Geometry: final body of the model. Coordinates: model frame, mm. A direction names the side the tool comes from. Coordinates: 2 decimals unless noted, no trailing zeros. Write each loop counter-clockwise with the first axis right and the second up, starting at its lowest first coordinate (ties: lowest second). Pieces come first, ordered by that corner, then holes. Notation, with made-up numbers: M 79.5,-26.75 L 113.5,-26.75 A7 ccw 113.5,-17.75 Z; hole C 62.25,10.5 d3. An arc over 180 degrees is marked long. Write item = value, one per line. Start each with the question number.
Item 1: Ray query, L1, parallel to Z at x = -27, y = -110.45; L2, parallel to Y at x = -227, z = 8.5; L3, parallel to Y at x = -419.5, z = 7.5. Return the intervals inside material, ascending. Write a range as [from, to].
Item 2: Reachability of faces 1 (the cylindrical face through (-30.23, 110.79, 18.79)), 2 (the flat face through (-62, -126.75, 25)), 3 (the flat face through (-214.22, 184.18, 24.65)) from +Z, -Z, +X, -X, +Y, -Y: full face, straight path, thin tool, end or side. Return the list, or none.
Item 3: First-contact query: pin 1 Ø6.5 at (y, z) = (-112, 17) entering from +X; pin 2 Ø12.5 at (x, z) = (-27, 25) entering from +Y; pin 3 Ø12 at (x, z) = (-290, 36.5) entering from -Y. Flat tips, straight axial feed; report the tip coordinate or a pass-through.
Item 4: Pull-direction query (Y, two-part tool) for faces 4 (the flat face through (-62, 126.75, 25)), 5 (the flat face through (-56, 120.75, 25)), 6 (the flat face through (-286.95, -242.43, 24.65)), 7 (the cylindrical face through (-23.77, -123.79, 18.79)); classes: +Y half, -Y half, draft (parallel to the pull), parting line (faces both ways), or undercut.
Item 5: Section B-B on y = 267. Output: boundary loops of the cut face in (x, z).
Item 6: Section A-A on x = -266. Output: boundary loops of the cut face in (y, z).
from build123d import *

# Parameters (mm, degrees)
PAD_DEPTH           = 50
PAD001_DEPTH        = 50
SKETCH015_R         = 6
POCKET005_DEPTH     = 10
LINEARPATTERN_COUNT = 4
LINEARPATTERN_PITCH = 130
PAD007_DEPTH        = 10
CHAMFER_SIZE        = 5
SKETCH016_R         = 7
POCKET_DEPTH        = 20
SKETCH017_R         = 7
POCKET006_DEPTH     = 20


with BuildPart() as part:
    # Sketch → Pad (new body)
    with BuildSketch(Plane.XY):
        with BuildLine():
            Line((-447.593833, 354.914912), (19.501599, 27.85117))
            ThreePointArc((34, 0), (30.158368, 15.699453), (19.501599, 27.85117))
            Line((28, 0), (34, 0))
            ThreePointArc((28, 0), (24.836303, 12.928961), (16.06014, 22.936257))
            Line((16.06014, 22.936257), (-451.035292, 350))
            Line((-451.035292, 350), (-447.593833, 354.914912))
        make_face()
    extrude(amount=PAD_DEPTH)

    # Sketch001 → Pad001 (join)
    with BuildSketch(Plane.XY):
        Polygon((-95, 107.75), (-103.568888, 113.75), (0, 113.75), (0, 107.75), align=None)
        Polygon((-113.431112, 120.75), (-122, 126.75), (0, 126.75), (0, 120.75), align=None)
    extrude(amount=PAD001_DEPTH)

    # Sketch015 → Pocket005 (cut)
    with BuildSketch(Plane(origin=(22.943057, 32.766082, 0), x_dir=(-0.819152, 0.573576, 0), z_dir=(0.573576, 0.819152, 0))):
        with Locations((454.477006, 25)):
            Circle(SKETCH015_R)
    pocket005 = extrude(amount=-POCKET005_DEPTH, mode=Mode.SUBTRACT)

    # LinearPattern: Pocket005 ×4
    with Locations(*[Vector(0.819152, -0.573576, 0) * (i * LINEARPATTERN_PITCH) for i in range(1, LINEARPATTERN_COUNT)]):
        add(pocket005, mode=Mode.SUBTRACT)

    # Sketch001 → Pad007 (join)
    with BuildSketch(Plane.XY):
        Polygon((-95, 107.75), (-103.568888, 113.75), (0, 113.75), (0, 107.75), align=None)
        Polygon((-113.431112, 120.75), (-122, 126.75), (0, 126.75), (0, 120.75), align=None)
    extrude(amount=PAD007_DEPTH)

    # Mirrored: part across XZ


with BuildPart() as part_1:
    add(part.part)
    add(part.part.mirror(Plane.XZ))

    # Chamfer
    chamfer_edges = [part_1.edges().sort_by_distance(p)[0] for p in [
        (0, -110.75, 50),
        (0, -123.75, 50),
        (0, -123.75, 0),
        (0, -110.75, 0),
        (0, 123.75, 50),
        (0, 110.75, 50),
        (0, 110.75, 0),
        (0, 123.75, 0),
    ]]
    chamfer(chamfer_edges, length=CHAMFER_SIZE)

    # Sketch016 (on Face21 of Chamfer) → Pocket (cut)
    with BuildSketch(Plane.XZ.offset(126.75)):
        with Locations((-27, 25)):
            Circle(SKETCH016_R)
    extrude(amount=-POCKET_DEPTH, mode=Mode.SUBTRACT)

    # Sketch017 (on Face1 of Pocket) → Pocket006 (cut)
    with BuildSketch(Plane(origin=(0, 126.75, 0), x_dir=(-1, 0, 0), z_dir=(0, 1, 0))):
        with Locations((27, 25)):
            Circle(SKETCH017_R)
    extrude(amount=-POCKET006_DEPTH, mode=Mode.SUBTRACT)


solid = part_1.part
Responses:
q1.L1 = [0, 18], [32, 50]
q1.L2 = [-200.45, -193.13], [193.13, 200.45]
q1.L3 = [-335.24, -327.92], [327.92, 335.24]
q2.face_1 = +Y
q2.face_2 = +Z, -Z, +X, -Y
q2.face_3 = +Z, -Z, -X
q3.pin_1 = 0
q3.pin_2 = 62.98
q3.pin_3 = -248.77
q4.face_4 = +Y half
q4.face_5 = undercut
q4.face_6 = -Y half
q4.face_7 = draft
q5.outline = M -332.5,0 L -322.04,0 L -322.04,50 L -332.5,50 Z
q6.outline = M -227.76,0 L -220.44,0 L -220.44,50 L -227.76,50 Z; M 220.44,0 L 227.76,0 L 227.76,50 L 220.44,50 Z
